Read the model definition and answer for the solid it produces. Units are mm, in the model's axes. Round coordinates to 2 decimals unless told otherwise and drop trailing zeros. Write each loop counter-clockwise with the first axis right and the second up, starting at its lowest first coordinate (ties: lowest second). Pieces come first, ordered by that corner, then holes.
from build123d import *

# Parameters (mm, degrees)
F0_R     = 25
F1_DEPTH = 80
F3_T     = -0.8
F2_R     = 13.75
F4_DEPTH = 25


with BuildPart() as f1:
    # F0 (on Top) → F1 (new body)
    with BuildSketch(Plane.XY):
        Circle(F0_R)
    extrude(amount=F1_DEPTH)

    # F3
    f3_openings = [f1.faces().sort_by_distance(p)[0] for p in [
        (0, 0, 80),
    ]]
    offset(amount=F3_T, openings=f3_openings)

    # F2 (on face) → F4 (cut)
    with BuildSketch(Plane(origin=(0, 0, 0), x_dir=(1, 0, 0), z_dir=(0, 0, -1))):
        Circle(F2_R)
    extrude(amount=-F4_DEPTH, mode=Mode.SUBTRACT)


solid = f1.part
Q1. Straight lines are drawn through the part: probe 1 along Y at (x, z) = (0, 42); probe 2 along X at (y, z) = (-17.5, 63); probe 3 along Z at (x, y) = (17.5, 0). For each, find the intervals that lie inside material, in ascending order.
Verdict:
probe 1: y = -25 to -24.2, 24.2 to 25
probe 2: x = -17.85 to -16.71, 16.71 to 17.85
probe 3: z = 0 to 0.8
Q2. Section A-A (y = 0) is taken. Determine the outline of the cut face in (x, z).
Verdict:
outline: (-25, 0) - (-13.75, 0) - (-13.75, 0.8) - (-24.2, 0.8) - (-24.2, 80) - (-25, 80) - close; (13.75, 0) - (25, 0) - (25, 80) - (24.2, 80) - (24.2, 0.8) - (13.75, 0.8) - close
Q3. Section D-D (x = 15.5) is taken. Determine the outline of the cut face in (y, z).
Verdict:
outline: (-19.62, 0) - (19.62, 0) - (19.62, 80) - (18.58, 80) - (18.58, 0.8) - (-18.58, 0.8) - (-18.58, 80) - (-19.62, 80) - close
Q4. Flat-ended cylindrical pins translate along their axes: pin 1 Ø8 at (y, z) = (18.5, 39.5) entering from +X; pin 2 Ø4 at (x, z) = (-13.5, 33.5) entering from +Y; pin 3 Ø10 at (y, z) = (17, 53.5) entering from -X; pin 4 Ø1.5 at (x, y) = (-14, 4) entering from -Z. Find the tip coordinate at first contact, or state that the pin passes through.
Verdict:
pin 1: stops at x = 20.37
pin 2: stops at y = 22.2
pin 3: stops at x = -21.93
pin 4: stops at z = 0
Q5. Determine the mould class of faces 1 (the cylindrical face through (-2.981, 13.423, 0.394)), 2 (the cylindrical face through (23.846, 7.509, 39.44)), 3 (the flat face through (11, -11, 0)) for opening direction X: pulls with the +X half, pulls with the -X half, needs draft (parallel to the pull), parting line crosses it, or undercut.
Verdict:
face 1: undercut
face 2: parting line crosses it
face 3: needs draft
Q6. Section C-C (z = 61.5) is taken. Determine the outline of the cut face in (x, y), then the cut area to 3 significant figures.
Verdict:
outline: circle Ø50 at (0, 0); hole circle Ø48.4 at (0, 0)
area: 124 mm2
